Job drawing, mm, ordinate dimensions from the low corner. One solid piece. A direction names the side the tool comes from. Give positions to 0.01 mm unless a question says otherwise; leave off trailing zeros. Loops run counter-clockwise (first coordinate to the right, second up) from the corner with the lowest first, then second, coordinate; pieces in that order, holes last. Notation, with made-up numbers: (56, -36) - (104, -36) arc R11 ccw to (104, -29) - close; hole circle Ø4 at (-33, 16.25). An arc over 180 degrees is marked (long way). Use a Markdown table: item, result.
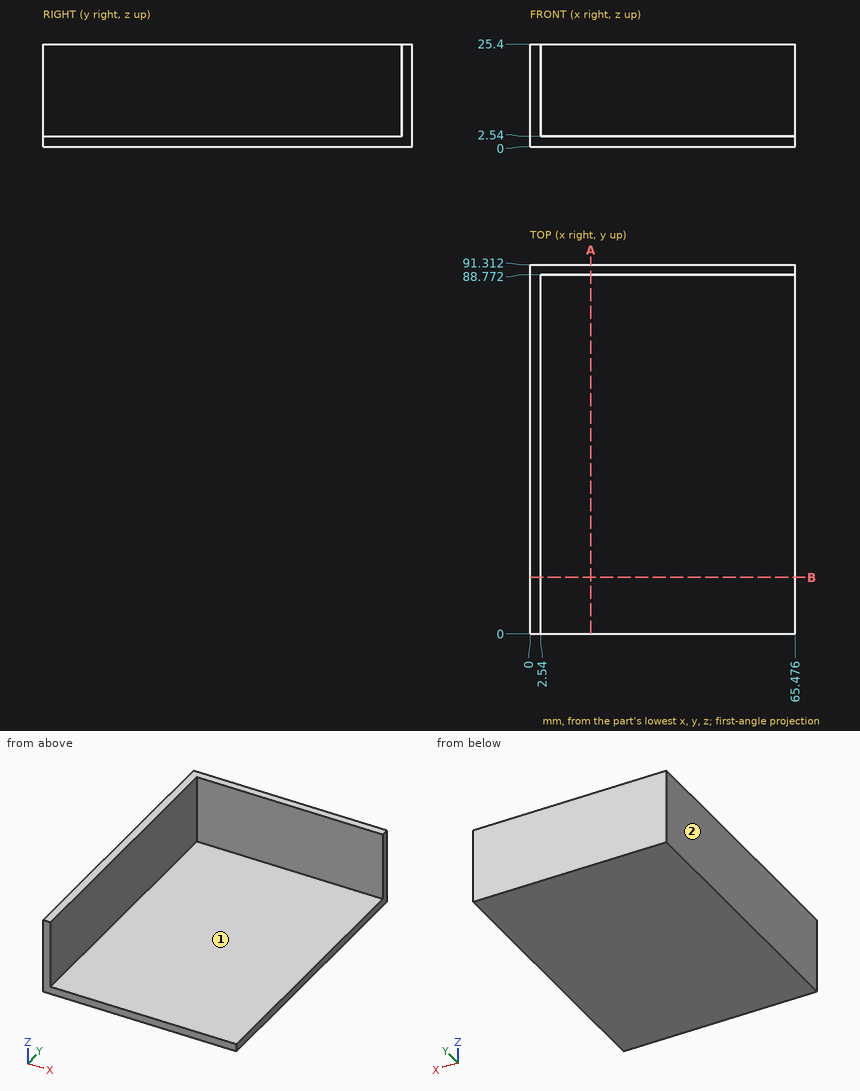
(1) Drill centre lines: probe 1 along Z at (x, y) = (16, 20.5); probe 2 along Y at (x, z) = (6.5, 15.25). Where is each one in solid material? Low to high. Write a range as [from, to].
Computed:
| item | result |
|---|---|
| probe 1 | [0, 2.54] |
| probe 2 | [88.77, 91.31] |
(2) Pin check, flat tips, straight feed: P1, Ø4, axis at x = 26, z = 5, coming from the -Y side; P2, Ø7, axis at y = 29, z = 15.5, coming from the +X side; P3, Ø10, axis at x = 57, y = 13, coming from the +Z side. Stop position of each tip, or through.
Computed:
| item | result |
|---|---|
| P1 | y = 88.77 |
| P2 | x = 2.54 |
| P3 | z = 2.54 |
(3) 3-axis set-ups, long thin cutter, end or side, ignore diameter. For the marked faces 1 and 2: which of +Z, -Z, +X, -X, +Y, -Y reach the whole face in a straight line?
Computed:
| item | result |
|---|---|
| face 1 | +Z, +X, -Y |
| face 2 | +Z, -Z, -X, +Y, -Y |
(4) Slice it at A-A, the plane x = 15. Write the cut outline in (y, z).
Computed:
| item | result |
|---|---|
| outline | (0, 0) - (91.31, 0) - (91.31, 25.4) - (88.77, 25.4) - (88.77, 2.54) - (0, 2.54) - close |
(5) Slice it at B-B, the plane y = 14. Write the cut outline in (x, z), plus the area to 3 significant figures.
Computed:
| item | result |
|---|---|
| outline | (0, 0) - (65.48, 0) - (65.48, 2.54) - (2.54, 2.54) - (2.54, 25.4) - (0, 25.4) - close |
| area | 224 mm² |
